Geometry check sheet. Reference: the model listing, model coordinates, mm. A direction names the side the tool comes from. Coordinates: 2 decimals unless noted, no trailing zeros. Loops run counter-clockwise (first coordinate to the right, second up) from the corner with the lowest first, then second, coordinate; pieces in that order, holes last.
from build123d import *

# Parameters (mm, degrees)
SKETCH1_R           = 2
SKETCH1_R_2         = 2.5
BOSS_EXTRUDE1_DEPTH = 5


with BuildPart() as part:
    # Sketch1 → Boss-Extrude1 (new body)
    with BuildSketch(Plane.XY):
        Polygon((-24.218289086, 78.115044248), (-24.218289086, 38.115044248), (5.781710914, 38.115044248), (5.781710914, -75.884955752), (-24.218289086, -75.884955752), (-24.218289086, -115.884955752), (45.781710914, -115.884955752), (45.781710914, 78.115044248), align=None)
        with Locations((25.781710914, -18.884955752)):
            Circle(SKETCH1_R, mode=Mode.SUBTRACT)
        with Locations((-6.718289086, -107.285805209)):
            Circle(SKETCH1_R_2, mode=Mode.SUBTRACT)
        with Locations(Location((28.281710914, -107.285805209, 0), (0, 0, 180))):
            Circle(SKETCH1_R_2, mode=Mode.SUBTRACT)
        with Locations((28.281710914, 69.515893704)):
            Circle(SKETCH1_R_2, mode=Mode.SUBTRACT)
        with Locations(Location((-6.718289086, 69.515893704, 0), (0, 0, 180))):
            Circle(SKETCH1_R_2, mode=Mode.SUBTRACT)
    extrude(amount=BOSS_EXTRUDE1_DEPTH)


solid = part.part
(1) Sectioned sample at C-C on y = -51.5. Record the cut outline in (x, z), and give its area (3 significant figures).
Findings:
outline: (5.78, 0) - (45.78, 0) - (45.78, 5) - (5.78, 5) - close
area: 200 mm2
(2) Sectioned sample at A-A on x = -0.5. Record the cut outline in (y, z), and give its area (3 significant figures).
Findings:
outline: (-115.88, 0) - (-75.88, 0) - (-75.88, 5) - (-115.88, 5) - close; (38.12, 0) - (78.12, 0) - (78.12, 5) - (38.12, 5) - close
area: 400 mm2
(3) Scan lines: L1, parallel to Y at x = 28, z = 1.3; L2, parallel to Y at x = -19.5, z = 2.55; L3, parallel to Y at x = 27, z = 3.8. Record each from-to range of solid material in increasing order.
Findings:
L1: y = -115.88 to -109.77, -104.8 to 67.03, 72 to 78.12
L2: y = -115.88 to -75.88, 38.12 to 78.12
L3: y = -115.88 to -109.43, -105.14 to -20.47, -17.3 to 67.37, 71.66 to 78.12
(4) Sectioned sample at B-B on z = 3.55. Record the cut outline in (x, y), and give its area (3 significant figures).
Findings:
outline: (-24.22, -115.88) - (45.78, -115.88) - (45.78, 78.12) - (-24.22, 78.12) - (-24.22, 38.12) - (5.78, 38.12) - (5.78, -75.88) - (-24.22, -75.88) - close; hole circle Ø5 at (-6.72, -107.29); hole circle Ø5 at (-6.72, 69.52); hole circle Ø4 at (25.78, -18.88); hole circle Ø5 at (28.28, -107.29); hole circle Ø5 at (28.28, 69.52)
area: 10,100 mm2
(5) Access from +Z, -Z, +X, -X, +Y, -Y to the whole of each face (thin tool, end or side, straight path). Record for faces 1 (the flat face through (-9, 38.115, 2)), 2 (the flat face through (45.782, -20, 2)).
Findings:
face 1: +Z, -Z, -X
face 2: +Z, -Z, +X, +Y, -Y
(6) Draft check along X on faces 3 (the flat face through (18, -18, 5)), 4 (the flat face through (-24.218, 58, 2)), 5 (the cylindrical face through (30.59, 68.56, 2.46)). Enter one of: +X half, -X half, draft (parallel to the pull), parting line (faces both ways), or undercut.
Findings:
face 3: draft
face 4: -X half
face 5: undercut
(7) Gauge pin test, flat ends, axial feed: pin 1 Ø1 at (y, z) = (9.5, 0.5) entering from -X; pin 2 Ø6.5 at (x, y) = (28.28, -107.29) entering from -Z. Record the tip position at first contact, or that the pin passes through.
Findings:
pin 1: stops at x = 5.78
pin 2: stops at z = 0
